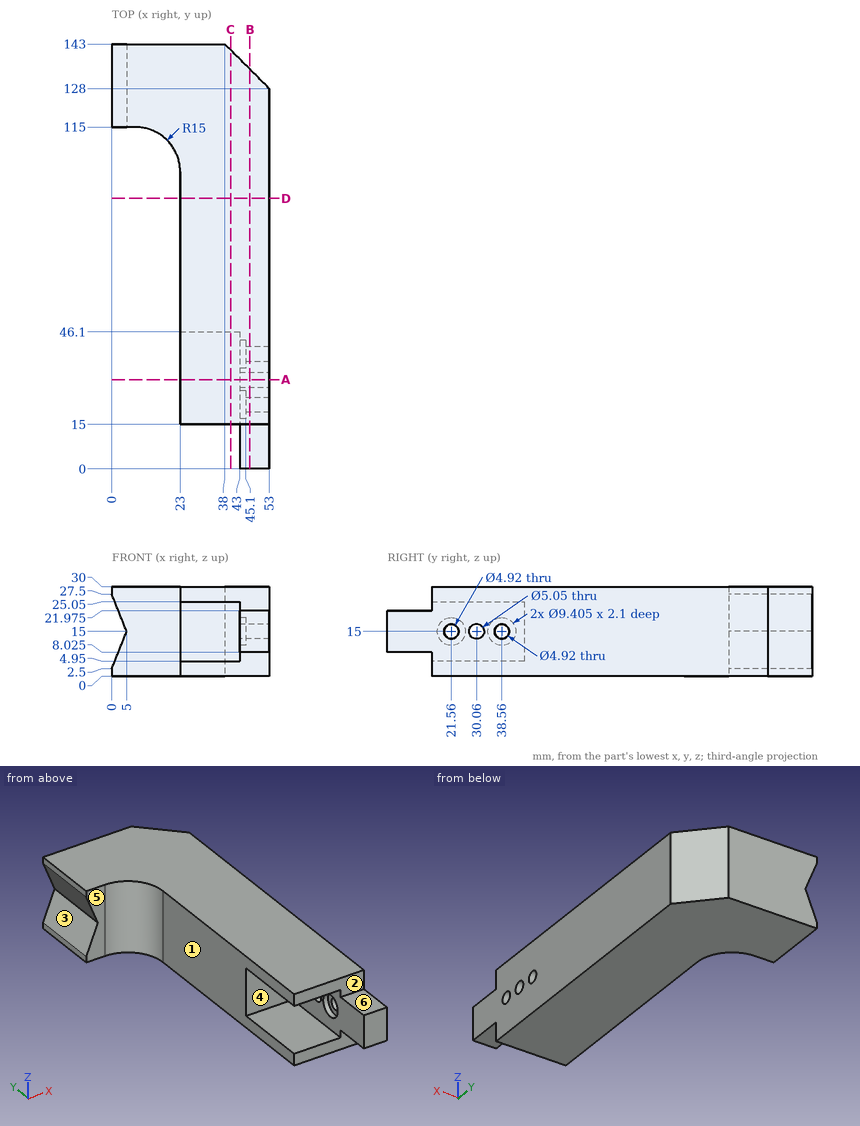
Input: dimensioned drawing with shaded views. Units: mm. Origin: part minimum x, y, z. A direction names the side the tool comes from. Coordinates: 2 decimals unless noted, no trailing zeros. Loops run counter-clockwise (first coordinate to the right, second up) from the corner with the lowest first, then second, coordinate; pieces in that order, holes last. Notation, with made-up numbers: (60.25, 58) -> (114.25, 58) arc R22 cw to (114.25, 76) -> close; hole circle Ø11 at (51, 17.25). An arc over 180 degrees is marked (long way). One line per item, written item: value. Start each with the question number.
Q1. Line query: line 1 along Z through (x, y) = (34.5, 27.5); line 2 along Y through (x, z) = (50.75, 15) (3 decimals); line 3 along Z through (x, y) = (51, 21.56). Output: solid intervals per line, ascending.
Q2. Set-up query: the marked faces 1, 2 and 3. Return all of +Z, -Z, +X, -X, +Y, -Y with unobstructed straight access to the full face (end or side cutting, diameter ignored); none if empty.
Q3. Section query D-D, the plane y = 91. Return the cut outline in (x, z), and give its area (3 significant figures).
Q4. Section query A-A, the plane y = 30.06. Return the cut outline in (x, z) (3 decimals), and give its area (4 significant figures).
Q5. Section query C-C, the plane x = 40. Return the cut outline in (y, z), and give its area (3 significant figures).
Q6. Mould query, pull axis Z, two halves, no side actions, for the marked faces 4, 5 and 6. Classes: pulls with the +Z half, pulls with the -Z half, needs draft (parallel to the pull), parting line crosses it, or undercut.
Q7. Contact query for flat-ended pins moving along their axis: P1, Ø4, axis at x = 2.5, z = 9.5, coming from the -Y side; P2, Ø2, axis at x = 35, y = 61, coming from the -Z side; P3, Ø4, axis at y = 21.56, z = 15, coming from the +X side (3 decimals); P4, Ø10, axis at x = 24, z = 24.5, coming from the -Y side. Output: stop coordinate, or through.
Q8. Section query B-B, the plane x = 46.5. Return the cut outline in (y, z) (3 decimals), and give its area (3 significant figures).
Results:
1. line 1: 0 to 4.95, 25.05 to 30
1. line 2: 0 to 19.1, 24.02 to 27.535, 32.585 to 36.1, 41.02 to 130.25
1. line 3: 0 to 12.54, 17.46 to 30
2. face 1: +Z, -Z, -X, -Y
2. face 2: +Z, +X, -X, -Y
2. face 3: -X, +Y, -Y
3. outline: (23, 0) -> (53, 0) -> (53, 30) -> (23, 30) -> close
3. area: 900 mm^2
4. outline: (23, 0) -> (53, 0) -> (53, 12.475) -> (43, 12.475) -> (43, 4.95) -> (23, 4.95) -> close; (23, 25.05) -> (43, 25.05) -> (43, 17.525) -> (53, 17.525) -> (53, 30) -> (23, 30) -> close
4. area: 447.5 mm^2
5. outline: (15, 0) -> (141, 0) -> (141, 30) -> (15, 30) -> (15, 25.05) -> (46.1, 25.05) -> (46.1, 4.95) -> (15, 4.95) -> close
5. area: 3,150 mm^2
6. face 4: undercut
6. face 5: needs draft
6. face 6: pulls with the +Z half
7. P1: y = 115
7. P2: z = 0
7. P3: through
7. P4: y = 15
8. outline: (0, 8.025) -> (15, 8.025) -> (15, 0) -> (134.5, 0) -> (134.5, 30) -> (15, 30) -> (15, 21.975) -> (0, 21.975) -> close; hole circle Ø4.92 at (21.56, 15); hole circle Ø5.05 at (30.06, 15); hole circle Ø4.92 at (38.56, 15)
8. area: 3,740 mm^2
